Design review of the part built by this model. Coordinates are the model's own, in mm. A direction names the side the tool comes from. Give positions to 0.01 mm unless a question says otherwise; leave off trailing zeros. Loops run counter-clockwise (first coordinate to the right, second up) from the corner with the lowest first, then second, coordinate; pieces in that order, holes last. Notation, with made-up numbers: (84, 2.5) - (104, 2.5) arc R17 cw to (104, 11.5) - close; hole circle Ø6 at (19.25, 67). An arc over 180 degrees is marked (long way). Write each question's results on one line, items separated by ' | '.
```python
from build123d import *

# Parameters (mm, degrees)
BOSS_EXTRUDE1_DEPTH = 50
SKETCH5_R           = 3.5
SKETCH5_R_2         = 1.5
BOSS_EXTRUDE2_DEPTH = 50
SKETCH6_R           = 1.5
CUT_EXTRUDE1_DEPTH  = 10
CUT_EXTRUDE2_START  = -10
SKETCH7_R           = 1.5
CUT_EXTRUDE2_DEPTH  = 10


with BuildPart() as part:
    # Sketch1 → Boss-Extrude1 (new body)
    with BuildSketch(Plane(origin=(0, 0, 0), x_dir=(1, 0, 0), z_dir=(0, 1, 0))):
        with BuildLine():
            Line((-2, 32), (-2, 0.828427125))
            Line((-2, 0.828427125), (-8.485281374, -5.656854249))
            ThreePointArc((-8.485281374, -5.656854249), (-8.485281374, -8.485281374), (-5.656854249, -8.485281374))
            Line((-5.656854249, -8.485281374), (2, -0.828427125))
            Line((2, -0.828427125), (2, 32))
            ThreePointArc((2, 32), (0, 34), (-2, 32))
        make_face()
    extrude(amount=BOSS_EXTRUDE1_DEPTH)

    # Sketch5 → Boss-Extrude2 (add, through all)
    # profile 1 of 2: a face of its own
    with BuildSketch(Plane(origin=(0, 0, 0), x_dir=(-1, 0, 0), z_dir=(0, -1, 0))):
        with Locations((1.5, 24.171572875)):
            Circle(SKETCH5_R)
        with Locations((1.5, 24.171572875)):
            Circle(SKETCH5_R_2, mode=Mode.SUBTRACT)
    # profile 2 of 2: a face of its own
    with BuildSketch(Plane(origin=(0, 0, 0), x_dir=(-1, 0, 0), z_dir=(0, -1, 0))):
        with Locations((4.01040764, -1.889087297)):
            Circle(SKETCH5_R)
        with Locations((4.01040764, -1.889087297)):
            Circle(SKETCH5_R_2, mode=Mode.SUBTRACT)
    extrude(amount=-BOSS_EXTRUDE2_DEPTH)

    # Sketch6 → Cut-Extrude1 (cut)
    with BuildSketch(Plane(origin=(0, 0, 0), x_dir=(-1, 0, 0), z_dir=(0, -1, 0))):
        with Locations(Location((4.01040764, -1.889087297, 0), (0, 0, 90))):
            Circle(SKETCH6_R)
        with Locations(Location((1.5, 24.171572875, 0), (0, 0, 90))):
            Circle(SKETCH6_R)
    extrude(amount=-CUT_EXTRUDE1_DEPTH, mode=Mode.SUBTRACT)

    # Sketch7 → Cut-Extrude2 (cut)
    with BuildSketch(Plane(origin=(0, 50, 0), x_dir=(1, 0, 0), z_dir=(0, 1, 0)).offset(CUT_EXTRUDE2_START)):
        with Locations(Location((-4.01040764, -1.889087297, 0), (0, 0, 90))):
            Circle(SKETCH7_R)
        with Locations(Location((-1.5, 24.171572875, 0), (0, 0, 90))):
            Circle(SKETCH7_R)
    extrude(amount=CUT_EXTRUDE2_DEPTH, mode=Mode.SUBTRACT)


solid = part.part
```
Item 1: Tool access review of faces 1 (the face through (-4.91, 24.65, 0.69)), 2 (the face through (-2, 25, -24)), 3 (the face through (-7.64, 24.65, 4.81)), 4 (the face through (-1, 10, -24)), 5 (the face through (-2, 25, -30)): name each direction out of +Z, -Z, +X, -X, +Y, -Y from which nothing blocks a thin tool from reaching the whole face with its end or side.
Output values:
face 1: none | face 2: +Y, -Y | face 3: -X, +Y, -Y | face 4: -Y | face 5: -Z, -X, +Y, -Y
Item 2: Clearance check with flat-ended pins moving along their axes: P1, Ø4, axis at x = -2.5, y = 33, coming from the +Z side; P2, Ø2.5, axis at x = -1.5, z = -24.17, coming from the +Y side; P3, Ø4, axis at x = 0, z = -0.5, coming from the -Y side; P4, Ø2.5, axis at y = 28.5, z = -24.5, coming from the -X side. State where each tip first meets the part, or that it passes through.
Output values:
P1: stops at z = 7.33 | P2: stops at y = 40 | P3: stops at y = 0 | P4: stops at x = -5
Item 3: We need section D-D on z = -7.5. Give the boundary of the cut face in (x, y), then the cut area to 3 significant figures.
Output values:
outline: (-2, 0) - (2, 0) - (2, 50) - (-2, 50) - close | area: 200 mm²
Item 4: We need section A-A on y = 8. Give the boundary of the cut face in (x, z), then the cut area to 3 significant figures.
Output values:
outline: (-8.49, 5.66) - (-6.81, 3.99) arc R3.5 ccw to (-2, -0.98) - (-2, -20.71) arc R3.5 ccw to (-2, -27.64) - (-2, -32) arc R2 ccw to (2, -32) - (2, 0.83) - (-5.66, 8.49) arc R2 ccw to start; hole circle Ø3 at (-4.01, 1.89); hole circle Ø3 at (-1.5, -24.17) | area: 198 mm²
Item 5: We need section B-B on z = 1.5. Give the boundary of the cut face in (x, y), then the cut area to 3 significant figures.
Output values:
outline: (-7.49, 0) - (-5.46, 0) - (-5.46, 50) - (-7.49, 50) - close; (-4.33, 10) - (-2.56, 10) - (-2.56, 0) - (1.33, 0) - (1.33, 50) - (-2.56, 50) - (-2.56, 40) - (-4.33, 40) - close | area: 349 mm²
Item 6: We need section C-C on y = 36. Give the boundary of the cut face in (x, z).
Output values:
outline: (-8.49, 5.66) - (-6.81, 3.99) arc R3.5 ccw to (-2, -0.98) - (-2, -20.71) arc R3.5 ccw to (-2, -27.64) - (-2, -32) arc R2 ccw to (2, -32) - (2, 0.83) - (-5.66, 8.49) arc R2 ccw to start; hole (-5.36, 2.54) arc R1.5 ccw to (-3.36, 0.54) - close; hole (-2, -25.59) - (-2, -22.76) arc R1.5 ccw to start
Item 7: Wall thickness on probe 1 along X at (y, z) = (4, -24); probe 2 along Z at (x, y) = (-0.75, 41); probe 3 along X at (y, z) = (47, -16.5): over which ranges is each line inside the solid? List them lowest first.
Output values:
probe 1: x = -5 to -2.99, -0.01 to 2 | probe 2: z = -33.85 to -25.47, -22.87 to 3.58 | probe 3: x = -2 to 2
